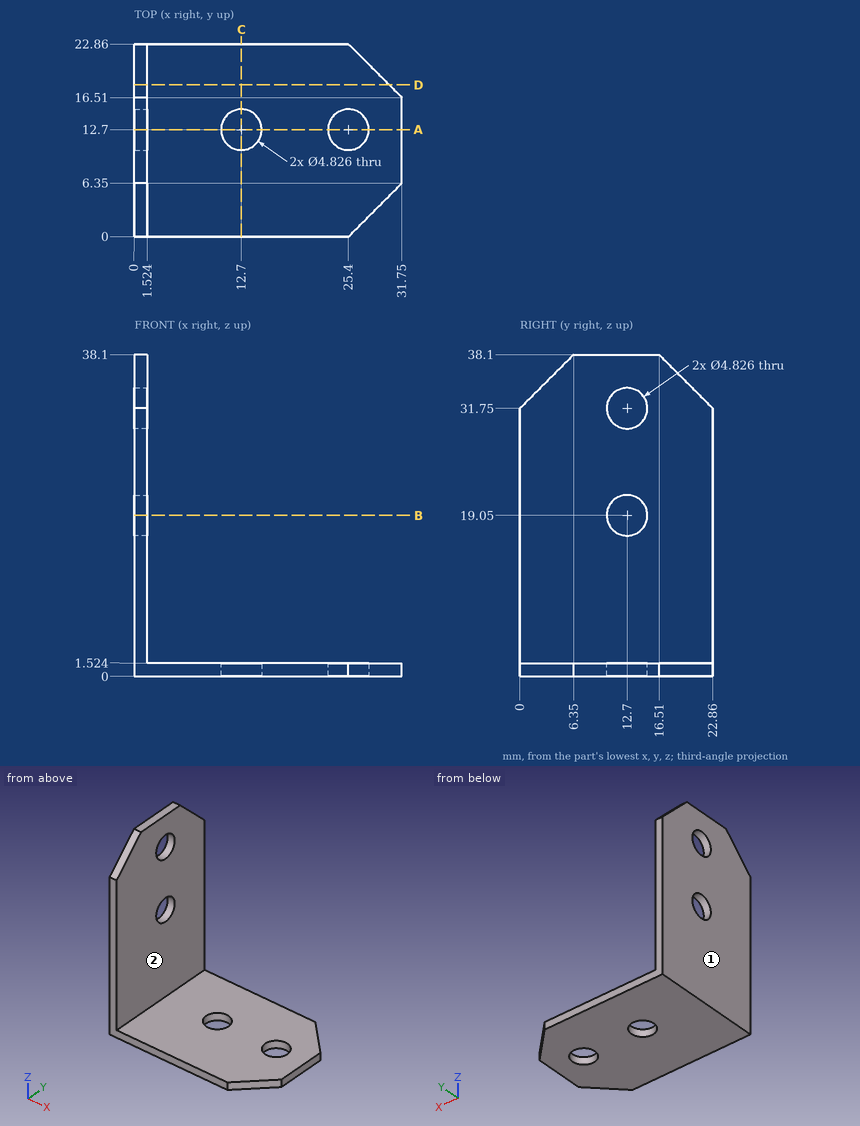
Here's the drawing with two shaded views (mm, measured from the low corner). I have some questions. A direction names the side the tool comes from. Give positions to 0.01 mm unless a question says otherwise; leave off trailing zeros. Loops run counter-clockwise (first coordinate to the right, second up) from the corner with the lowest first, then second, coordinate; pieces in that order, holes last. Notation, with made-up numbers: M 52,59.25 L 91,59.25 A26 cw 91,75.25 Z; hole C 85,2.25 d4. An arc over 180 degrees is marked long. Use one line per item in the form item = value. Start each with the question number.
(1) I want a section at D-D, the plane y = 18. Write out the boundary of the cut face in (x, z), and give its area (3 significant figures).
(2) I want a section at B-B, the plane z = 19.05. Write out the boundary of the cut face in (x, y).
(3) I'm going to push flat-ended pins straight in: P1, Ø7, axis at x = 12, y = 13.5, coming from the +Z side; P2, Ø7, axis at y = 11, z = 21.5, coming from the +X side. Where does each tip first touch, or does it pass through?
(4) On a 3-axis mill with a long thin cutter (end or side, diameter ignored), from which of +Z, -Z, +X, -X, +Y, -Y can I reach the whole of each face in a straight line? I mean the marked faces 1 and 2. Say none if no direction works.
(5) Please list where these lines run through material, in increasing order: line 1 (X direction, y = 10.5, z = 5); line 2 (Y direction, x = 25, z = 1).
(6) I want a section at A-A, the plane y = 12.7. Write out the boundary of the cut face in (x, z), and give its area (3 significant figures).
(7) I want a section at C-C, the plane x = 12.7. Write out the boundary of the cut face in (y, z), and give its area (3 significant figures).
Worked out:
q1.outline = M 0,0 L 30.26,0 L 30.26,1.52 L 1.52,1.52 L 1.52,36.61 L 0,36.61 Z
q1.area = 99.6 mm²
q2.outline = M 0,0 L 1.52,0 L 1.52,10.29 L 0,10.29 Z; M 0,15.11 L 1.52,15.11 L 1.52,22.86 L 0,22.86 Z
q3.P1 = 1.52
q3.P2 = 1.52
q4.face_1 = +Z, -Z, -X, +Y, -Y
q4.face_2 = +Z, +X, +Y, -Y
q5.line_1 = 0 to 1.52
q5.line_2 = 0 to 10.32, 15.08 to 22.86
q6.outline = M 0,0 L 10.29,0 L 10.29,1.52 L 1.52,1.52 L 1.52,16.64 L 0,16.64 Z; M 0,21.46 L 1.52,21.46 L 1.52,29.34 L 0,29.34 Z; M 0,34.16 L 1.52,34.16 L 1.52,38.1 L 0,38.1 Z; M 15.11,0 L 22.99,0 L 22.99,1.52 L 15.11,1.52 Z; M 27.81,0 L 31.75,0 L 31.75,1.52 L 27.81,1.52 Z
q6.area = 74.7 mm²
q7.outline = M 0,0 L 10.29,0 L 10.29,1.52 L 0,1.52 Z; M 15.11,0 L 22.86,0 L 22.86,1.52 L 15.11,1.52 Z
q7.area = 27.5 mm²
